Check sheet for the modelled part. Datum: model origin and axes. Units: mm. A direction names the side the tool comes from. Give positions to 0.01 mm unless a question says otherwise; leave off trailing zeros. Order: outer loops, then holes, each group sorted by start corner. A loop starts at its lowest first (then second) coordinate and runs counter-clockwise, first axis right, second up.
```python
from build123d import *

# Parameters (mm, degrees)
BOSS_EXTRUDE2_DEPTH                  = 3
F_13_64_0_20313_DIAMETER_HOLE1_D     = 5.159502
F_13_64_0_20313_DIAMETER_HOLE1_DEPTH = 3
CUT_EXTRUDE1_DEPTH                   = 4
FILLET2_R                            = 2
FILLET3_R                            = 2
FILLET4_R                            = 2
FILLET5_R                            = 2
F_3_0MM_DOWEL_HOLE1_D                = 3
F_3_0MM_DOWEL_HOLE1_DEPTH            = 3
F_10_0MM_DOWEL_HOLE1_D               = 10
F_10_0MM_DOWEL_HOLE1_DEPTH           = 3
F_10_0MM_DOWEL_HOLE2_D               = 10
F_10_0MM_DOWEL_HOLE2_DEPTH           = 3
F_3_0MM_DOWEL_HOLE2_D                = 3
F_3_0MM_DOWEL_HOLE2_DEPTH            = 3


with BuildPart() as part:
    # Sketch3 → Boss-Extrude2 (new body)
    with BuildSketch(Plane(origin=(0, 0, 0), x_dir=(1, 0, 0), z_dir=(0, 1, 0))):
        Polygon((146.917568262, 30.566233816), (11.506619665, 165.977182413), (-68.75, 165.977182413), (-165.977182413, 68.75), (-165.977182413, -11.506619665), (-30.566233816, -146.917568262), (49.690385849, -146.917568262), (146.917568262, -49.690385849), align=None)
    extrude(amount=BOSS_EXTRUDE2_DEPTH)

    # 13/64 (0.20313) Diameter Hole1
    with Locations(Plane(origin=(0, 0, 0), x_dir=(-1, 0, 0), z_dir=(0, -1, 0))):
        with Locations((39.029807033, 9.528212544), (9.528212544, -19.970192881), (-19.970192881, 9.531401607), (9.531401607, 39.029807033)):
            Hole(F_13_64_0_20313_DIAMETER_HOLE1_D / 2, depth=F_13_64_0_20313_DIAMETER_HOLE1_DEPTH)

    # Sketch12 → Cut-Extrude1 (cut, through all)
    with BuildSketch(Plane.XZ):
        Polygon((-36.04631137, -36.04631137), (-39.581845276, -32.510777464), (-53.7239809, -46.652913088), (-46.652913088, -53.7239809), (-32.510777464, -39.581845276), align=None)
    extrude(amount=-CUT_EXTRUDE1_DEPTH, mode=Mode.SUBTRACT)

    # Fillet2
    fillet2_edges = [part.edges().sort_by_distance(p)[0] for p in [
        (-39.581845276, 1.5, -32.510777464),
    ]]
    fillet(fillet2_edges, radius=FILLET2_R)

    # Fillet3
    fillet3_edges = [part.edges().sort_by_distance(p)[0] for p in [
        (-32.510777464, 1.5, -39.581845276),
    ]]
    fillet(fillet3_edges, radius=FILLET3_R)

    # Fillet4
    fillet4_edges = [part.edges().sort_by_distance(p)[0] for p in [
        (-53.7239809, 1.5, -46.652913088),
    ]]
    fillet(fillet4_edges, radius=FILLET4_R)

    # Fillet5
    fillet5_edges = [part.edges().sort_by_distance(p)[0] for p in [
        (-46.652913088, 1.5, -53.7239809),
    ]]
    fillet(fillet5_edges, radius=FILLET5_R)

    # Ø3.0mm Dowel Hole1
    with Locations(Plane(origin=(0, 0, 0), x_dir=(-1, 0, 0), z_dir=(0, -1, 0))):
        with Locations((-76.383242623, -90.45627663), (-90.453906961, -76.384091118), (-77.79601145, -63.7275639), (-63.725347112, -77.799749412), (-19.512076016, -125.867568262), (-19.512076016, -107.967568262), (0.387923984, -125.867568262), (0.387923984, -107.967568262), (63.695294959, -58.704128358), (76.351822177, -71.362023869), (90.42400769, -57.291359531), (77.767480471, -44.63346402), (144.927182413, 38.571690168), (127.027182413, 38.571690168), (127.027182413, 18.671690168), (144.927182413, 18.671690168), (96.855625588, 82.78717805), (82.784961264, 96.859363576), (95.442856787, 109.515890782), (109.513521111, 95.443705257), (18.671690168, 144.927182413), (18.671690168, 127.027182413), (38.571690168, 127.027182413), (38.571690168, 144.927182413), (-58.70786632, 63.693078171), (-71.364393538, 76.350973682), (-44.635680808, 77.763742509), (-57.292208026, 90.42163802), (-125.867568262, -19.512076016), (-107.967568262, -19.512076016), (-107.967568262, 0.387923984), (-125.867568262, 0.387923984)):
            Hole(F_3_0MM_DOWEL_HOLE1_D / 2, depth=F_3_0MM_DOWEL_HOLE1_DEPTH)

    # Ø10.0mm Dowel Hole1
    with Locations(Plane(origin=(0, 3, 0), x_dir=(1, 0, 0), z_dir=(0, 1, 0))):
        with Locations((-135.977182413, 28.621690168), (-96.149241188, 96.151534416), (-28.621690168, 135.977182413), (58.000037173, 77.057358096), (116.917568262, -9.562076016)):
            Hole(F_10_0MM_DOWEL_HOLE1_D / 2, depth=F_10_0MM_DOWEL_HOLE1_DEPTH)

    # Ø10.0mm Dowel Hole2
    with Locations(Plane(origin=(0, 3, 0), x_dir=(1, 0, 0), z_dir=(0, 1, 0))):
        with Locations((9.562076016, -116.917568262), (77.089627036, -77.091920265), (-77.059651324, -57.997743944)):
            Hole(F_10_0MM_DOWEL_HOLE2_D / 2, depth=F_10_0MM_DOWEL_HOLE2_DEPTH)

    # Ø3.0mm Dowel Hole2
    with Locations(Plane(origin=(0, 0, 0), x_dir=(-1, 0, 0), z_dir=(0, -1, 0))):
        with Locations((62.825395525, -43.770951614), (-43.770951614, -43.765781374), (62.830565765, 62.825395525), (-43.765781374, 62.830565765)):
            Hole(F_3_0MM_DOWEL_HOLE2_D / 2, depth=F_3_0MM_DOWEL_HOLE2_DEPTH)


solid = part.part
```
Q1. Sectioned sample at A-A, the plane x = -136. Record the cut outline in (y, z), plus the area to 3 significant figures.
Q2. Go/stop test with flat-tipped pins: P1, Ø4, axis at x = -62.83, z = 43.77, coming from the +Y side; P2, Ø2.5, axis at x = 90.45, z = 76.38, coming from the +Y side (3 decimals). Record where each tip stops, or that it passes through.
Q3. Material ranges on line 1 (Z direction, x = 44.5, y = 1.2); line 2 (Z direction, x = 109, y = 2.65); line 3 (Z direction, x = -62.5, y = 1.35), recorded low to high.
Q4. Draft check along Z on faces 3 (the cylindrical face through (-27.971, 1.479, -140.935)), 4 (the cylindrical face through (-140.746, 1.479, -30.124)), 5 (the flat face through (-12, 3, -12)), 6 (the flat face through (80.16, 1.479, -97.324)). Enter one of: pulls with the +Z half, pulls with the -Z half, needs draft (parallel to the pull), parting line crosses it, or undercut.
Q5. Tool access check on faces 1 (the flat face through (-99.22, 1.479, 78.264)), 2 (the flat face through (-46.57, 1.48, -39.5)). Record the directions out of +Z, -Z, +X, -X, +Y, -Y that give a thin tool (end or side, any length) a straight path to the whole face; none if there is none.
Q6. Sectioned sample at B-B, the plane y = 1.8. Count the separate pieces of the cut face and the enclosed holes in it, plus the area to 3 significant figures.
Filled in:
1. outline: (0, -98.73) - (3, -98.73) - (3, -33.62) - (0, -33.62) - close; (0, -23.62) - (3, -23.62) - (3, 41.48) - (0, 41.48) - close
1. area: 391 mm2
2. P1: stops at y = 3
2. P2: passes through
3. line 1: z = -132.98 to -79.26, -76.27 to -64.14, -61.52 to 42.45, 45.08 to 146.92
3. line 2: z = -68.48 to -1.48, 0.7 to 18.42, 20.6 to 87.61
3. line 3: z = -165.98 to -64.29, -61.36 to 42.31, 45.24 to 57.8, 59.61 to 114.98
4. face 3: undercut
4. face 4: undercut
4. face 5: needs draft
4. face 6: pulls with the -Z half
5. face 1: +Z, -X, +Y, -Y
5. face 2: +Y, -Y
6. separate pieces: 1
6. enclosed holes: 49
6. area: 69,000 mm2
